Check sheet for the modelled part. Datum: model origin and axes. Units: mm. A direction names the side the tool comes from. Give positions to 0.01 mm unless a question says otherwise; leave off trailing zeros. Write each loop counter-clockwise with the first axis right and the second up, starting at its lowest first coordinate (ties: lowest second). Pieces come first, ordered by that corner, then holes. Notation, with made-up numbers: M 42,23 L 66,23 A15 cw 66,41 Z; hole C 61,-26.75 d2. An arc over 180 degrees is marked long. Use CSV: the item, a comma, the result in double quotes. Start each with the question number.
1. Cross-section at C-C, the plane z = 103. Enter the section's corners in (x, y), and give its area (3 significant figures).
2. Cross-section at B-B, the plane x = -24. Enter the section's corners in (y, z).
3. Cross-section at A-A, the plane x = 4. Enter the section's corners in (y, z), and give its area (3 significant figures).
4. Access from +Z, -Z, +X, -X, +Y, -Y to the whole of each face (thin tool, end or side, straight path). Record for faces 4 (the face through (30, -31, 32)), 5 (the face through (15, 26, 8.295)), 6 (the face through (15.21, -65.81, -28.7)).
5. Scan lines: line 1 (Z direction, x = 24.5, y = -54); line 2 (Z direction, x = 10.5, y = -58); line 3 (X direction, y = 46, z = 1). Record each from-to range of solid material in increasing order.
6. Depth check by flat-ended pin: P1, Ø8, axis at x = 36, z = -23.5, coming from the +Y side; P2, Ø24, axis at x = 8, z = 54, coming from the +Y side; P3, Ø24, axis at x = 9.5, z = 45, coming from the -Y side. Enter the tip coordinate at first touch or a pass-through.
7. Cross-section at D-D, the plane y = 56.5. Enter the section's corners in (x, z).
8. Mould release check, pull along Y, two halves, no side actions. Record for faces 1 (the face through (14.79, -21.67, 125.44)), 2 (the face through (14.024, -144.837, -3.733)), 3 (the face through (57, -117.666, -29)): +Y half, -Y half, draft (parallel to the pull), parting line (faces both ways), or undercut.
from build123d import *

# Parameters (mm, degrees)
F1_W      = 140
F1_H      = 160
F2_DEPTH  = 30
F3_R      = 10
F4_W      = 90
F4_H      = 120
F5_DEPTH  = 30.001
F6_R      = 10
F7_D      = 11
F8_R      = 7.5
F9_DEPTH  = 100
F11_R     = 50
F12_DEPTH = 2
F13_R     = 45
F13_R_2   = 7.5
F14_DEPTH = 4
F15_R     = 47.5
F16_DEPTH = 4


with BuildPart() as f2:
    # F1 (on Right) → F2 (new body)
    with BuildSketch(Plane.YZ):
        with Locations((1.3344958425, 48.294539011)):
            Rectangle(F1_W, F1_H)
    extrude(amount=F2_DEPTH)

    # F3
    f3_edges = [f2.edges().sort_by_distance(p)[0] for p in [
        (15, -68.665504, 128.294539),
        (15, -68.665504, -31.705461),
    ]]
    fillet(f3_edges, radius=F3_R)

    # F4 (on face) → F5 (cut, through all)
    with BuildSketch(Plane.YZ.offset(30)):
        with Locations((26.3344958425, 68.294539011)):
            Rectangle(F4_W, F4_H)
    extrude(amount=-F5_DEPTH, mode=Mode.SUBTRACT)

    # F6
    f6_edges = [f2.edges().sort_by_distance(p)[0] for p in [
        (15, -18.665504, 128.294539),
        (15, -18.665504, 8.294539),
        (15, 71.334496, 8.294539),
        (15, 71.334496, -31.705461),
    ]]
    fillet(f6_edges, radius=F6_R)

    # F7 (through all)
    with Locations(Plane(origin=(0, 0, 0), x_dir=(0, 1, 0), z_dir=(-1, 0, 0))):
        with Locations((-53.3879697323, -118.0560608581), (-53.3879697323, 11.9439391419), (41.6120302677, 11.9439391419)):
            Hole(F7_D / 2)

    # F8 (on face) → F9 (join)
    with BuildSketch(Plane.XZ.offset(68.6655041575)):
        with Locations((15, -11.168804951)):
            Circle(F8_R)
    extrude(amount=F9_DEPTH)

    # F11 (on offset) → F12 (join)
    with BuildSketch(Plane.XZ.offset(111.6655041575)):
        with Locations((15, -11.168804951)):
            Circle(F11_R)
    extrude(amount=F12_DEPTH)

    # F13 (on face) → F14 (join)
    with BuildSketch(Plane.XZ.offset(113.6655041575)):
        with Locations((15, -11.168804951)):
            Circle(F13_R)
        with Locations((15, -11.168804951)):
            Circle(F13_R_2, mode=Mode.SUBTRACT)
    extrude(amount=F14_DEPTH)

    # F15 (on face) → F16 (join)
    with BuildSketch(Plane.XZ.offset(117.6655041575)):
        with Locations((15, -11.168804951)):
            Circle(F15_R)
    extrude(amount=F16_DEPTH)


solid = f2.part
Worked answers:
1,outline,"M 0,-68.67 L 30,-68.67 L 30,-18.67 L 0,-18.67 Z"
1,area,"1,500 mm^2"
2,outline,"M -121.67,-38.28 L -117.67,-38.28 L -117.67,-33.62 L -113.67,-33.62 L -113.67,-42.46 L -111.67,-42.46 L -111.67,20.12 L -113.67,20.12 L -113.67,11.28 L -117.67,11.28 L -117.67,15.95 L -121.67,15.95 Z"
3,outline,"M -121.67,-57.38 L -117.67,-57.38 L -117.67,-54.8 L -113.67,-54.8 L -113.67,-59.94 L -111.67,-59.94 L -111.67,37.61 L -113.67,37.61 L -113.67,32.47 L -117.67,32.47 L -117.67,35.04 L -121.67,35.04 Z; M -68.67,-21.71 A10 ccw -58.67,-31.71 L 61.33,-31.71 A10 ccw 71.33,-21.71 L 71.33,-1.71 A10 ccw 61.33,8.29 L -8.67,8.29 A10 cw -18.67,18.29 L -18.67,118.29 A10 ccw -28.67,128.29 L -58.67,128.29 A10 ccw -68.67,118.29 Z; hole C -53.39,-11.94 d11; hole C -53.39,118.06 d11; hole C 41.61,-11.94 d11"
3,area,"12,100 mm^2"
4,face 4,"+Z, -Z, +X, +Y"
4,face 5,"+Z, +X, -X, +Y"
4,face 6,"-Z, +X, -X"
5,line 1,"z = -31.71 to -17.41, -6.48 to 112.59, 123.52 to 128.29"
5,line 2,"z = -31.71 to -14.94, -8.95 to 115.06, 121.05 to 128.29"
5,line 3,"x = 0 to 30"
6,P1,"stops at y = -111.67"
6,P2,"stops at y = -18.67"
6,P3,"stops at y = -121.67"
7,outline,"M 0,-31.71 L 30,-31.71 L 30,8.29 L 0,8.29 Z"
8,face 1,"+Y half"
8,face 2,"draft"
8,face 3,"undercut"
